```python
from build123d import *

# Parameters (mm, degrees)
SKETCH1_W                       = 225.16353247
SKETCH1_H                       = 204.4
BOSS_EXTRUDE1_DEPTH             = 15
HOLE1_D                         = 6
HOLE1_CBORE_D                   = 11
HOLE1_CBORE_DEPTH               = 5
M5X0_8_TAPPED_HOLE1_D           = 4.2
M5X0_8_TAPPED_HOLE1_ON_FACE_2_D = 4.2
CUT_EXTRUDE1_DEPTH              = 5
M6X1_0_TAPPED_HOLE1_D           = 5
HOLE2_D                         = 5
HOLE2_CBORE_D                   = 11
HOLE2_CBORE_DEPTH               = 5
CUT_EXTRUDE2_DEPTH              = 5
CHAMFER1_SIZE                   = 40
SKETCH16_W                      = 53
SKETCH16_H                      = 35.620178703
SKETCH16_H_2                    = 37.110089351
CUT_EXTRUDE3_DEPTH              = 1
SKETCH16_3_W                    = 53
SKETCH16_3_H                    = 130.179821297
CUT_EXTRUDE4_DEPTH              = 5
CUT_EXTRUDE5_DEPTH              = 256.382465743
CUT_EXTRUDE6_DEPTH              = 5
FILLET1_R                       = 10
OLDSPINDLEMOUNTM8HOLES_D        = 7


with BuildPart() as part:
    # Sketch1 → Boss-Extrude1 (new body)
    with BuildSketch(Plane.XY):
        with Locations((81.081766235, -63.6)):
            Rectangle(SKETCH1_W, SKETCH1_H)
    extrude(amount=BOSS_EXTRUDE1_DEPTH)

    # Hole1 (through all)
    with Locations(Plane(origin=(-26.5, 20, 15), x_dir=(1, 0, 0), z_dir=(0, 0, 1))):
        with Locations((0, 0), (53, -40), (53, 0), (0, -40), (53, -82.2), (53, -122.2), (0, -82.2), (0, -122.2), (162.16353247, 0), (162.16353247, -40), (215.16353247, 0), (215.16353247, -82.2), (215.16353247, -40), (162.16353247, -122.2), (162.16353247, -82.2), (215.16353247, -122.2), (90.031766235, -24.020178703), (90.031766235, -48.220178703), (125.131766235, -48.220178703), (125.131766235, -24.020178703)):
            CounterBoreHole(HOLE1_D / 2, HOLE1_CBORE_D / 2, HOLE1_CBORE_DEPTH)

    # M5x0.8 Tapped Hole1 (through all)
    with Locations(Plane(origin=(162.164010883, -82.200361066, 15), x_dir=(1, 0, 0), z_dir=(0, 0, 1))):
        with Locations((0, 0), (-162.164010883, 0.000361066), (-0.000478413, 82.200361066), (-0.000478413, 0.000361066), (-162.164010883, 82.200361066)):
            Hole(M5X0_8_TAPPED_HOLE1_D / 2)

    # M5x0.8 Tapped Hole1 on face 2 (through all)
    with Locations(Plane(origin=(0, 0, 0), x_dir=(-1, 0, 0), z_dir=(0, 0, -1))):
        with Locations((0, 0)):
            Hole(M5X0_8_TAPPED_HOLE1_ON_FACE_2_D / 2)

    # Sketch9 → Cut-Extrude1 (cut)
    with BuildSketch(Plane.XY.offset(15)):
        with BuildLine():
            Line((-31.5, 14.5), (-26.5, 14.5))
            ThreePointArc((-26.5, 14.5), (-29.470514841, 15.371172764), (-31.5, 17.708712153))
            Line((-31.5, 17.708712153), (-31.5, 14.5))
        make_face()
        with BuildLine():
            ThreePointArc((-31.5, 22.291287847), (-29.470514841, 24.628827236), (-26.5, 25.5))
            Line((-26.5, 25.5), (-31.5, 25.5))
            Line((-31.5, 25.5), (-31.5, 22.291287847))
        make_face()
        with BuildLine():
            Line((-26.5, -14.5), (-31.5, -14.5))
            Line((-31.5, -14.5), (-31.5, -17.708712153))
            ThreePointArc((-31.5, -17.708712153), (-29.470514841, -15.371172764), (-26.5, -14.5))
        make_face()
        with BuildLine():
            Line((-31.5, -25.5), (-26.5, -25.5))
            ThreePointArc((-26.5, -25.5), (-29.470514841, -24.628827236), (-31.5, -22.291287847))
            Line((-31.5, -22.291287847), (-31.5, -25.5))
        make_face()
        with BuildLine():
            Line((-26.5, -56.7), (-31.5, -56.7))
            Line((-31.5, -56.7), (-31.5, -59.908712153))
            ThreePointArc((-31.5, -59.908712153), (-29.470514841, -57.571172764), (-26.5, -56.7))
        make_face()
        with BuildLine():
            Line((-31.5, -67.7), (-26.5, -67.7))
            ThreePointArc((-26.5, -67.7), (-29.470514841, -66.828827236), (-31.5, -64.491287847))
            Line((-31.5, -64.491287847), (-31.5, -67.7))
        make_face()
        with BuildLine():
            Line((-26.5, -96.7), (-31.5, -96.7))
            Line((-31.5, -96.7), (-31.5, -99.908712153))
            ThreePointArc((-31.5, -99.908712153), (-29.470514841, -97.571172764), (-26.5, -96.7))
        make_face()
        with BuildLine():
            Line((-31.5, -107.7), (-26.5, -107.7))
            ThreePointArc((-26.5, -107.7), (-29.470514841, -106.828827236), (-31.5, -104.491287847))
            Line((-31.5, -104.491287847), (-31.5, -107.7))
        make_face()
        with BuildLine():
            ThreePointArc((193.66353247, -104.491287847), (191.634047311, -106.828827236), (188.66353247, -107.7))
            Line((188.66353247, -107.7), (193.66353247, -107.7))
            Line((193.66353247, -107.7), (193.66353247, -104.491287847))
        make_face()
        with BuildLine():
            Line((193.66353247, -99.908712153), (193.66353247, -96.7))
            Line((193.66353247, -96.7), (188.66353247, -96.7))
            ThreePointArc((188.66353247, -96.7), (191.634047311, -97.571172764), (193.66353247, -99.908712153))
        make_face()
        with BuildLine():
            ThreePointArc((193.66353247, -64.491287847), (191.634047311, -66.828827236), (188.66353247, -67.7))
            Line((188.66353247, -67.7), (193.66353247, -67.7))
            Line((193.66353247, -67.7), (193.66353247, -64.491287847))
        make_face()
        with BuildLine():
            Line((193.66353247, -59.908712153), (193.66353247, -56.7))
            Line((193.66353247, -56.7), (188.66353247, -56.7))
            ThreePointArc((188.66353247, -56.7), (191.634047311, -57.571172764), (193.66353247, -59.908712153))
        make_face()
        with BuildLine():
            ThreePointArc((193.66353247, -22.291287848), (191.634047311, -24.628827236), (188.66353247, -25.5))
            Line((188.66353247, -25.5), (193.66353247, -25.5))
            Line((193.66353247, -25.5), (193.66353247, -22.291287848))
        make_face()
        with BuildLine():
            Line((193.66353247, -17.708712153), (193.66353247, -14.5))
            Line((193.66353247, -14.5), (188.66353247, -14.5))
            ThreePointArc((188.66353247, -14.5), (191.634047311, -15.371172764), (193.66353247, -17.708712153))
        make_face()
        with BuildLine():
            ThreePointArc((193.66353247, 17.708712152), (191.634047311, 15.371172764), (188.66353247, 14.5))
            Line((188.66353247, 14.5), (193.66353247, 14.5))
            Line((193.66353247, 14.5), (193.66353247, 17.708712152))
        make_face()
        with BuildLine():
            Line((193.66353247, 25.5), (188.66353247, 25.5))
            ThreePointArc((188.66353247, 25.5), (191.634047311, 24.628827236), (193.66353247, 22.291287847))
            Line((193.66353247, 22.291287847), (193.66353247, 25.5))
        make_face()
    extrude(amount=-CUT_EXTRUDE1_DEPTH, mode=Mode.SUBTRACT)

    # M6x1.0 Tapped Hole1 (through all)
    with Locations(Plane(origin=(16.081766235, -96.8, 15), x_dir=(1, 0, 0), z_dir=(0, 0, 1))):
        with Locations((0, 0), (130, 0), (130, -60), (0, -60)):
            Hole(M6X1_0_TAPPED_HOLE1_D / 2)

    # Hole2 (through all)
    with Locations(Plane(origin=(16.081766235, -105.8, 15), x_dir=(1, 0, 0), z_dir=(0, 0, 1))):
        with Locations((0, 0), (0, -42), (130, 0), (130, -42)):
            CounterBoreHole(HOLE2_D / 2, HOLE2_CBORE_D / 2, HOLE2_CBORE_DEPTH)

    # Sketch15 → Cut-Extrude2 (cut)
    with BuildSketch(Plane.XY.offset(15)):
        with BuildLine():
            Line((24.703704526, -97.001603846), (14.285470762, -100.601603846))
            ThreePointArc((14.285470762, -100.601603846), (19.273190282, -101.320623643), (21.581766235, -105.8))
            ThreePointArc((21.581766235, -105.8), (20.561142593, -108.991424047), (17.878061709, -110.998396154))
            Line((17.878061709, -110.998396154), (28.296295473, -107.398396154))
            ThreePointArc((28.296295473, -107.398396154), (21.301603846, -103.996295474), (24.703704526, -97.001603846))
        make_face()
        with BuildLine():
            Line((133.867236997, -107.398396154), (144.285470762, -110.998396154))
            ThreePointArc((144.285470762, -110.998396154), (140.883370081, -104.003704527), (147.878061709, -100.601603846))
            Line((147.878061709, -100.601603846), (137.459827944, -97.001603846))
            ThreePointArc((137.459827944, -97.001603846), (140.142908828, -99.008575953), (141.16353247, -102.2))
            ThreePointArc((141.16353247, -102.2), (138.854956517, -106.679376358), (133.867236997, -107.398396154))
        make_face()
    extrude(amount=-CUT_EXTRUDE2_DEPTH, mode=Mode.SUBTRACT)

    # Chamfer1
    chamfer1_edges = [part.edges().sort_by_distance(p)[0] for p in [
        (193.66353247, -165.8, 7.5),
        (-31.5, -165.8, 7.5),
    ]]
    chamfer(chamfer1_edges, length=CHAMFER1_SIZE)

    # Sketch16 → Cut-Extrude3 (cut)
    with BuildSketch(Plane(origin=(0, 0, 0), x_dir=(-1, 0, 0), z_dir=(0, 0, -1))):
        with Locations((-81.081766235, -17.810089352)):
            Rectangle(SKETCH16_W, SKETCH16_H)
        with Locations((-81.081766235, 20.044955325)):
            Rectangle(SKETCH16_W, SKETCH16_H_2)
    extrude(amount=-CUT_EXTRUDE3_DEPTH, mode=Mode.SUBTRACT)

    # Sketch16<3> → Cut-Extrude4 (cut)
    with BuildSketch(Plane(origin=(0, 0, 0), x_dir=(-1, 0, 0), z_dir=(0, 0, -1))):
        with Locations((-81.081766235, -100.710089352)):
            Rectangle(SKETCH16_3_W, SKETCH16_3_H)
    extrude(amount=-CUT_EXTRUDE4_DEPTH, mode=Mode.SUBTRACT)

    # Sketch16<4> → Cut-Extrude5 (cut, through all)
    with BuildSketch(Plane(origin=(0, 0, 0), x_dir=(-1, 0, 0), z_dir=(0, 0, -1))):
        Polygon((-54.581766235, 1.489910649), (-107.581766235, 1.489910649), (-107.581766235, 38.6), (-130.66353247, 38.6), (-130.66353247, 0), (-31.5, 0), (-31.5, 38.6), (-54.581766235, 38.6), align=None)
    extrude(amount=-CUT_EXTRUDE5_DEPTH, mode=Mode.SUBTRACT)


with BuildPart() as cut_extrude5_kept_piece:
    # of the separate pieces the step leaves, the one the design keeps (cut_extrude5_pieces_kept)
    add(part.part.solids().sort_by_distance((193.66353247, -125.8, 15))[0])

    # Sketch17 → Cut-Extrude6 (cut)
    with BuildSketch(Plane.XY.offset(15)):
        with BuildLine():
            Line((26.5, 25.5), (37.535291554, 25.5))
            ThreePointArc((37.535291554, 25.5), (43.035291554, 20), (37.535291554, 14.5))
            Line((37.535291554, 14.5), (26.5, 14.5))
            ThreePointArc((26.5, 14.5), (21, 20), (26.5, 25.5))
        make_face()
        with BuildLine():
            Line((58.031766235, -4.020178703), (58.031766235, 6.878958383))
            ThreePointArc((58.031766235, 6.878958383), (63.531766235, 12.378958383), (69.031766235, 6.878958383))
            Line((69.031766235, 6.878958383), (69.031766235, -4.020178703))
            ThreePointArc((69.031766235, -4.020178703), (63.531766235, -9.520178703), (58.031766235, -4.020178703))
        make_face()
        with BuildLine():
            Line((93.131766235, -4.020178703), (93.131766235, 8.238121163))
            ThreePointArc((93.131766235, 8.238121163), (98.631766235, 13.738121163), (104.131766235, 8.238121163))
            Line((104.131766235, 8.238121163), (104.131766235, -4.020178703))
            ThreePointArc((104.131766235, -4.020178703), (98.631766235, -9.520178703), (93.131766235, -4.020178703))
        make_face()
        with BuildLine():
            Line((135.66353247, 14.5), (124.67272757, 14.5))
            ThreePointArc((124.67272757, 14.5), (119.17272757, 20), (124.67272757, 25.5))
            Line((124.67272757, 25.5), (135.66353247, 25.5))
            ThreePointArc((135.66353247, 25.5), (141.16353247, 20), (135.66353247, 14.5))
        make_face()
    extrude(amount=-CUT_EXTRUDE6_DEPTH, mode=Mode.SUBTRACT)

    # Fillet1
    fillet1_edges = [cut_extrude5_kept_piece.edges().sort_by_distance(p)[0] for p in [
        (193.66353247, -125.8, 7.5),
        (8.5, -165.8, 7.5),
        (153.66353247, -165.8, 7.5),
        (-31.5, -125.8, 7.5),
        (31.5, 0, 7.5),
        (130.66353247, 38.6, 7.5),
        (31.5, 38.6, 7.5),
        (130.66353247, 0, 7.5),
        (-31.5, 38.6, 7.5),
        (193.66353247, 38.6, 7.5),
    ]]
    fillet(fillet1_edges, radius=FILLET1_R)

    # oldSpindleMountM8holes (through all)
    with Locations(Plane(origin=(31.581766235, -7.5, 15), x_dir=(1, 0, 0), z_dir=(0, 0, 1))):
        with Locations((0, 0), (0, -25), (99, 0), (99, -25)):
            Hole(OLDSPINDLEMOUNTM8HOLES_D / 2)


solid = cut_extrude5_kept_piece.part
```
The listing builds one solid part. Answer for the finished solid, in the listing's coordinates (mm). A direction names the side the tool comes from. Round coordinates to 2 decimals unless told otherwise and drop trailing zeros. Loops run counter-clockwise (first coordinate to the right, second up) from the corner with the lowest first, then second, coordinate; pieces in that order, holes last. Notation, with made-up numbers: (-39, -2) - (-23, -2) arc R23 cw to (-23, 6) - close; hole circle Ø2 at (36.5, -38). An arc over 180 degrees is marked (long way). Use one line per item in the form item = value. Start each with the question number.
1. Given pin 1 Ø4.5 at (x, z) = (99.5, 11) entering from +Y; pin 2 Ø1.5 at (y, z) = (-137.5, 13.5) entering from +X; pin 3 Ø2.5 at (x, z) = (-30, 13) entering from -Y, each flat-ended and moving along its own axis, determine where each tip first touches the part or whether it passes through.
2. For a pull along X with two mould halves and no side action, classify faces 1 (the face through (-11.3, -146, 7.4)), 2 (the face through (191, -25.5, 13)), 3 (the face through (143.697, -147.049, 4.93)) as pulls with the +X half, pulls with the -X half, needs draft (parallel to the pull), parting line crosses it, or undercut.
3. A tool of negligible diameter and unlimited length cuts with its end or side. For faces 4 (the face through (-29, -105, 10)), 5 (the face through (82, 0, 7)), 6 (the face through (101, -31, 10)), 7 (the face through (192, 20, 10)), from which of +Z, -Z, +X, -X, +Y, -Y can it reach the whole face along a straight path? Write none if from no direction.
4. The part is cut by section A-A on y = 20. Give the number of separate pieces and of enclosed holes in the cut face, then the cut area to 3 significant figures.
5. The part is cut by section C-C on y = -147.8. Determine the outline of the cut face in (x, z), then the cut area to 3 significant figures.
6. The part is cut by section B-B on x = 98.5. Determine the outline of the cut face in (y, z), then the cut area to 3 significant figures.
7. Consider line 1 (X direction, y = -96.5, z = 7); line 2 (X direction, y = -0.5, z = 8.5); line 3 (Y direction, x = 136, z = 13.5). Determine where each line is inside the solid, lowest interval first. Write a range as [from, to].
Geometry check:
q1.pin_1 = 0
q1.pin_2 = 182.71
q1.pin_3 = -128.55
q2.face_1 = pulls with the -X half
q2.face_2 = needs draft
q2.face_3 = undercut
q3.face_4 = +Z, -X
q3.face_5 = +Z, -Z, +Y
q3.face_6 = +Z
q3.face_7 = +Z, +X
q4.separate_pieces = 6
q4.enclosed_holes = 0
q4.area = 1,440 mm^2
q5.outline = (-9.5, 0) - (13.58, 0) - (13.58, 10) - (10.58, 10) - (10.58, 15) - (-9.5, 15) - close; (18.58, 0) - (54.58, 0) - (54.58, 5) - (107.58, 5) - (107.58, 0) - (143.58, 0) - (143.58, 10) - (140.58, 10) - (140.58, 15) - (21.58, 15) - (21.58, 10) - (18.58, 10) - close; (148.58, 0) - (171.66, 0) - (171.66, 15) - (151.58, 15) - (151.58, 10) - (148.58, 10) - close
q5.area = 2,240 mm^2
q6.outline = (-165.8, 5) - (-35.62, 5) - (-35.62, 1) - (-31.22, 1) - (-31.22, 10) - (-33.72, 10) - (-33.72, 15) - (-165.8, 15) - close; (-25.22, 1) - (-7.02, 1) - (-7.02, 10) - (-9.52, 10) - (-9.52, 15) - (-22.72, 15) - (-22.72, 10) - (-25.22, 10) - close; (-1.02, 1) - (0, 1) - (0, 10) - (-1.02, 10) - close
q6.area = 1,590 mm^2
q7.line_1 = [-31.5, 13.6], [18.56, 143.6], [148.56, 193.66]
q7.line_2 = [-31.5, -2.04], [2.04, 160.12], [164.2, 193.66]
q7.line_3 = [-165.8, -108.14], [-96.71, -67.69], [-56.71, -25.49], [-14.51, 14.51], [25.49, 37.45]
